from build123d import *

# Parameters (mm, degrees)
F1_DEPTH = 12
F2_DEPTH = 10
F3_SIZE  = 10
F4_R     = 3.25
F5_DEPTH = 4
F7_DEPTH = 10
F8_R     = 2.3


with BuildPart() as f1:
    # F0 (on Top) → F1 (new body)
    with BuildSketch(Plane.XY):
        Polygon((-8.1961524227, 4.7320508076), (-8.1961524227, -4.7320508076), (0, -9.4641016151), (8.1961524227, -4.7320508076), (8.1961524227, 4.7320508076), (0, 9.4641016151), align=None)
        Polygon((-5.1961524227, 3), (0, 6), (5.1961524227, 3), (5.1961524227, -3), (0, -6), (-5.1961524227, -3), align=None, mode=Mode.SUBTRACT)
    extrude(amount=F1_DEPTH)

    # F2 (add): a face of the model
    f2_faces = [f1.faces().sort_by_distance(p)[0] for p in [
        (8.1961524227, 0, 6),
    ]]
    extrude(f2_faces, amount=F2_DEPTH)

    # F3
    f3_edges = [f1.edges().sort_by_distance(p)[0] for p in [
        (18.196152, 0, 0),
    ]]
    chamfer(f3_edges, length=F3_SIZE)

    # F4 (on face) → F5 (join)
    with BuildSketch(Plane.XY.offset(12)):
        Polygon((0, 9.4641016151), (-8.1961524227, 4.7320508076), (-8.1961524227, -4.7320508076), (0, -9.4641016151), (8.1961524227, -4.7320508076), (18.1961524227, -4.7320508076), (18.1961524227, 4.7320508076), (8.1961524227, 4.7320508076), align=None)
        Polygon((-5.1961524227, -3), (-5.1961524227, 3), (0, 6), (5.1961524227, 3), (5.1961524227, -3), (0, -6), align=None, mode=Mode.SUBTRACT)
        Polygon((0, 6), (-5.1961524227, 3), (-5.1961524227, -3), (0, -6), (5.1961524227, -3), (5.1961524227, 3), align=None)
        Circle(F4_R, mode=Mode.SUBTRACT)
    extrude(amount=F5_DEPTH)

    # F6 (on face) → F7 (join)
    with BuildSketch(Plane.XY.offset(16)):
        with BuildLine():
            ThreePointArc((0, -3.5), (-3.5, 0), (0, 3.5))
            Line((0, 3.5), (18.1961524227, 3.5))
            Line((18.1961524227, 3.5), (18.1961524227, 4.7320508076))
            Line((18.1961524227, 4.7320508076), (8.1961524227, 4.7320508076))
            Line((8.1961524227, 4.7320508076), (4.0980762114, 7.0980762114))
            Line((4.0980762114, 7.0980762114), (-4.0980762114, 7.0980762114))
            Line((-4.0980762114, 7.0980762114), (-8.1961524227, 4.7320508076))
            Line((-8.1961524227, 4.7320508076), (-8.1961524227, -4.7320508076))
            Line((-8.1961524227, -4.7320508076), (-4.0980762114, -7.0980762114))
            Line((-4.0980762114, -7.0980762114), (4.0980762114, -7.0980762114))
            Line((4.0980762114, -7.0980762114), (8.1961524227, -4.7320508076))
            Line((8.1961524227, -4.7320508076), (18.1961524227, -4.7320508076))
            Line((18.1961524227, -4.7320508076), (18.1961524227, -3.5))
            Line((18.1961524227, -3.5), (0, -3.5))
        make_face()
    extrude(amount=F7_DEPTH)

    # F8
    f8_edges = [f1.edges().sort_by_distance(p)[0] for p in [
        (0, -7.098076, 16),
        (0, 7.098076, 16),
    ]]
    fillet(f8_edges, radius=F8_R)


solid = f1.part
Could you check a few things on this model? Use its own coordinates, in mm. A direction names the side the tool comes from. Give positions to 0.01 mm unless a question says otherwise; leave off trailing zeros. Order: outer loops, then holes, each group sorted by start corner. A loop starts at its lowest first (then second) coordinate and runs counter-clockwise, first axis right, second up. Notation, with made-up numbers: M -17,52 L 17,52 A16 cw 17,71 Z; hole C -3.75,70.5 d2. An arc over 180 degrees is marked long. One line per question, with ' | ' between items.
1. We'd pull the mould along X, two halves only. Please class faces 5 (the face through (-4, 4, 0)), 6 (the face through (5.196, 0, 6)), 7 (the face through (13.266, -0.066, 5.07)), 8 (the face through (2.6, 4.5, 5.9)): +X half, -X half, draft (parallel to the pull), parting line (faces both ways), or undercut.
Results:
face 5: draft | face 6: undercut | face 7: +X half | face 8: undercut
2. For faces 1 (the face through (0, -7.098, 22)), 2 (the face through (0, 7.098, 22)), 3 (the face through (-2.6, -4.5, 5.9)), 4 (the face through (13, 4.732, 16)), which set-ups out of +Z, -Z, +X, -X, +Y, -Y let a thin tool reach every point of the face, with its end or its side?
Results:
face 1: +Z, +X, -X, -Y | face 2: +Z, +X, -X, +Y | face 3: -Z | face 4: +Z, -Z, +X, +Y
3. I want a section at B-B (z = 11). List the corners of the cut face in (x, y) for me.
Results:
outline: M -8.2,-4.73 L 0,-9.46 L 8.2,-4.73 L 18.2,-4.73 L 18.2,4.73 L 8.2,4.73 L 0,9.46 L -8.2,4.73 Z; hole M -5.2,-3 L 0,-6 L 5.2,-3 L 5.2,3 L 0,6 L -5.2,3 Z
4. I'm going to push flat-ended pins straight in: pin 1 (6 mm diameter, centred on x = 2.5, y = 0, fed in from +Z); pin 2 (5 mm diameter, centred on x = 7, z = 11, fed in from -Y); pin 3 (4 mm diameter, centred on x = 3.5, z = 8, fed in from -Y); pin 4 (10.5 mm diameter, centred on x = 0, y = 0, fed in from +Z). Where does each tip first touch, or does it pass through?
Results:
pin 1: z = 16 | pin 2: y = -6.87 | pin 3: y = -8.6 | pin 4: z = 26
5. I want a section at A-A (y = 0). List the corners of the cut face in (x, z) for me.
Results:
outline: M -8.2,0 L -5.2,0 L -5.2,12 L -3.25,12 L -3.25,16 L -3.5,16 L -3.5,26 L -8.2,26 Z; M 3.25,12 L 5.2,12 L 5.2,0 L 8.2,0 L 18.2,10 L 18.2,16 L 3.25,16 Z
6. If I drill on line 1 (Y direction, x = 8.75, z = 24.5); line 2 (Z direction, x = -3.75, y = 3.5); line 3 (X direction, y = -0.75, z = 11), over which ranges is the centre line in solid material (lowest first)?
Results:
line 1: -4.73 to -3.5, 3.5 to 4.73 | line 2: 12 to 26 | line 3: -8.2 to -5.2, 5.2 to 18.2
7. I want a section at C-C (x = 13.5). List the corners of the cut face in (y, z) for me, and give its area (3 significant figures).
Results:
outline: M -4.73,5.3 L 4.73,5.3 L 4.73,26 L 3.5,26 L 3.5,16 L -3.5,16 L -3.5,26 L -4.73,26 Z | area: 126 mm²
8. I want a section at D-D (z = 7.5). List the corners of the cut face in (x, y) for me.
Results:
outline: M -8.2,-4.73 L 0,-9.46 L 8.2,-4.73 L 15.7,-4.73 L 15.7,4.73 L 8.2,4.73 L 0,9.46 L -8.2,4.73 Z; hole M -5.2,-3 L 0,-6 L 5.2,-3 L 5.2,3 L 0,6 L -5.2,3 Z
